Could you check a few things on this model? Use its own coordinates, in mm. A direction names the side the tool comes from. Round coordinates to 2 decimals unless told otherwise and drop trailing zeros. Loops run counter-clockwise (first coordinate to the right, second up) from the corner with the lowest first, then second, coordinate; pieces in that order, holes last. Notation, with made-up numbers: M 31.25,-29.75 L 87.25,-29.75 A25 ccw 87.25,-9.75 Z; hole C 87.5,81.25 d10. An arc over 180 degrees is marked long. Answer in a Markdown table with one row per item.
```python
from build123d import *

# Parameters (mm, degrees)
SKETCH_1_R      = 1.525
SKETCH_1_R_2    = 2.5
SKETCH_1_R_3    = 1.625
SKETCH_1_W      = 12.5
SKETCH_1_H      = 5
SKETCH_1_W_2    = 40
SKETCH_1_H_2    = 20
EXTRUDE_1_DEPTH = 5
FILLET_1_R      = 5


with BuildPart() as part:
    # 草图1 → 凸台-拉伸1 (new body)
    with BuildSketch(Plane(origin=(0, 0, 0), x_dir=(1, 0, 0), z_dir=(0, 1, 0))):
        with BuildLine():
            Line((41.868178549, 31.675), (158.5, 31.675))
            Line((158.5, 31.675), (158.5, -31.675))
            Line((158.5, -31.675), (41.868178549, -31.675))
            ThreePointArc((41.868178549, -31.675), (-52.5, 0), (41.868178549, 31.675))
        make_face()
        with Locations(Location((-33.55358156, 33.720895004, 0), (0, 0, 270))):
            Circle(SKETCH_1_R, mode=Mode.SUBTRACT)
        with Locations(Location((0, 0, 0), (0, 0, 270))):
            Circle(SKETCH_1_R_2, mode=Mode.SUBTRACT)
        with Locations(Location((82.254, 18.675, 0), (0, 0, 270))):
            Circle(SKETCH_1_R_3, mode=Mode.SUBTRACT)
        with Locations(Location((82.254, -8.825, 0), (0, 0, 270))):
            Circle(SKETCH_1_R_3, mode=Mode.SUBTRACT)
        with Locations(Location((135, 24.425, 0), (0, 0, 270))):
            Circle(SKETCH_1_R_3, mode=Mode.SUBTRACT)
        with Locations(Location((135, -24.425, 0), (0, 0, 90))):
            Circle(SKETCH_1_R_3, mode=Mode.SUBTRACT)
        with Locations(Location((33.720895004, 33.55358156, 0), (0, 0, 270))):
            Circle(SKETCH_1_R, mode=Mode.SUBTRACT)
        with Locations(Location((33.55358156, -33.720895004, 0), (0, 0, 270))):
            Circle(SKETCH_1_R, mode=Mode.SUBTRACT)
        with Locations(Location((-33.720895004, -33.55358156, 0), (0, 0, 270))):
            Circle(SKETCH_1_R, mode=Mode.SUBTRACT)
        with Locations((23.75, -20)):
            Rectangle(SKETCH_1_W, SKETCH_1_H, mode=Mode.SUBTRACT)
        with Locations((-23.75, 20)):
            Rectangle(SKETCH_1_W, SKETCH_1_H, mode=Mode.SUBTRACT)
        with Locations((0, 20)):
            Rectangle(SKETCH_1_W, SKETCH_1_H, mode=Mode.SUBTRACT)
        with Locations((23.75, 20)):
            Rectangle(SKETCH_1_W, SKETCH_1_H, mode=Mode.SUBTRACT)
        with Locations((0, -20)):
            Rectangle(SKETCH_1_W, SKETCH_1_H, mode=Mode.SUBTRACT)
        with Locations((-23.75, -20)):
            Rectangle(SKETCH_1_W, SKETCH_1_H, mode=Mode.SUBTRACT)
        with BuildLine():
            Line((-10, -30.25), (10, -30.25))
            ThreePointArc((10, -30.25), (15, -35.25), (10, -40.25))
            Line((10, -40.25), (-10, -40.25))
            ThreePointArc((-10, -40.25), (-15, -35.25), (-10, -30.25))
        make_face(mode=Mode.SUBTRACT)
        with BuildLine():
            Line((-10, 40.25), (10, 40.25))
            ThreePointArc((10, 40.25), (15, 35.25), (10, 30.25))
            Line((10, 30.25), (-10, 30.25))
            ThreePointArc((-10, 30.25), (-15, 35.25), (-10, 40.25))
        make_face(mode=Mode.SUBTRACT)
        with BuildLine():
            Line((48.183761531, 20.125053296), (48.183761531, -20.125053296))
            ThreePointArc((48.183761531, -20.125053296), (50, -21.941291765), (51.816238469, -20.125053296))
            Line((51.816238469, -20.125053296), (51.816238469, 20.125053296))
            ThreePointArc((51.816238469, 20.125053296), (50, 21.941291765), (48.183761531, 20.125053296))
        make_face(mode=Mode.SUBTRACT)
        with BuildLine():
            Line((68.183761531, 20.125053296), (68.183761531, -20.125053296))
            ThreePointArc((68.183761531, -20.125053296), (70, -21.941291765), (71.816238469, -20.125053296))
            Line((71.816238469, -20.125053296), (71.816238469, 20.125053296))
            ThreePointArc((71.816238469, 20.125053296), (70, 21.941291765), (68.183761531, 20.125053296))
        make_face(mode=Mode.SUBTRACT)
        with Locations((114.25, 0)):
            Rectangle(SKETCH_1_W_2, SKETCH_1_H_2, mode=Mode.SUBTRACT)
    extrude(amount=EXTRUDE_1_DEPTH)

    # 圆角1
    fillet_1_edges = [part.edges().sort_by_distance(p)[0] for p in [
        (94.25, 2.5, -10),
        (94.25, 2.5, 10),
        (134.25, 2.5, 10),
        (134.25, 2.5, -10),
        (41.868178549, 2.5, -31.675),
        (158.5, 2.5, -31.675),
        (158.5, 2.5, 31.675),
        (41.868178549, 2.5, 31.675),
    ]]
    fillet(fillet_1_edges, radius=FILLET_1_R)


solid = part.part
```
1) I want a section at A-A, the plane x = 104. Please give me the cut outline in (y, z) (3 decimals), plus the area to 3 significant figures.
Computed:
| item | result |
|---|---|
| outline | M 0,-31.675 L 5,-31.675 L 5,-10 L 0,-10 Z; M 0,10 L 5,10 L 5,31.675 L 0,31.675 Z |
| area | 217 mm² |
2) If we mould it in two halves opening along X, with no side actions, what happens to faces 4 (the face through (-52.47, 2.46, 1.8)), 5 (the face through (15, 2.46, -35.36)), 6 (the face through (100, 2, 31.675)), 7 (the face through (156.996, 2.535, -30.249))? For each: released by +X, released by -X, zero draft, split by the parting line, or undercut.
Computed:
| item | result |
|---|---|
| face 4 | split by the parting line |
| face 5 | undercut |
| face 6 | zero draft |
| face 7 | released by +X |
3) I want a section at D-D, the plane y = 3.65. State how many separate pieces and enclosed holes the cut face has, plus the area to 3 significant figures.
Computed:
| item | result |
|---|---|
| separate pieces | 1 |
| enclosed holes | 20 |
| area | 13,500 mm² |
4) Which directions (+Z, -Z, +X, -X, +Y, -Y) give clear straight access to the entire face, cutting with the end or side of a thin tool? Please do faces 1 (the face through (98, 2, -31.675)), 2 (the face through (-6.25, 2, 20)), 3 (the face through (42.13, 2.535, 32.163)).
Computed:
| item | result |
|---|---|
| face 1 | -Z, +X, +Y, -Y |
| face 2 | +Y, -Y |
| face 3 | +Z, +X, +Y, -Y |
5) Will these pins go through, and if not, where does the flat tip stop? P1, Ø2.5, axis at y = 3.5, z = -20, coming from the -X side; P2, Ø2.5, axis at x = 23.5, y = 3.5, coming from the +Z side; P3, Ø1, axis at x = -27.5, y = 3, coming from the +Z side (3 decimals); P4, Ø1.5, axis at x = 46.5, z = 20.5, coming from the -Y side.
Computed:
| item | result |
|---|---|
| P1 | stops at x = -49.04 |
| P2 | stops at z = 47.55 |
| P3 | stops at z = 45.025 |
| P4 | stops at y = 0 |
6) I want a section at C-C, the plane x = 0. Please give me the cut outline in (y, z).
Computed:
| item | result |
|---|---|
| outline | M 0,-52.5 L 5,-52.5 L 5,-40.25 L 0,-40.25 Z; M 0,-30.25 L 5,-30.25 L 5,-22.5 L 0,-22.5 Z; M 0,-17.5 L 5,-17.5 L 5,-2.5 L 0,-2.5 Z; M 0,2.5 L 5,2.5 L 5,17.5 L 0,17.5 Z; M 0,22.5 L 5,22.5 L 5,30.25 L 0,30.25 Z; M 0,40.25 L 5,40.25 L 5,52.5 L 0,52.5 Z |
7) I want a section at B-B, the plane z = 0. Please give me the cut outline in (x, y), plus the area to 3 significant figures.
Computed:
| item | result |
|---|---|
| outline | M -52.5,0 L -2.5,0 L -2.5,5 L -52.5,5 Z; M 2.5,0 L 48.18,0 L 48.18,5 L 2.5,5 Z; M 51.82,0 L 68.18,0 L 68.18,5 L 51.82,5 Z; M 71.82,0 L 94.25,0 L 94.25,5 L 71.82,5 Z; M 134.25,0 L 158.5,0 L 158.5,5 L 134.25,5 Z |
| area | 794 mm² |
8) I need wall thicknesses on line 1 (X direction, y = 1.7, z = -34.5); line 2 (Z direction, x = 9, y = 3.5); line 3 (X direction, y = 0.75, z = -15). Which ranges of each line are inside material? Lowest first, please.
Computed:
| item | result |
|---|---|
| line 1 | x = -39.57 to -34.86, -32.24 to -14.94, 14.94 to 32.53, 34.92 to 39.57 |
| line 2 | z = -51.72 to -40.25, -30.25 to 30.25, 40.25 to 51.72 |
| line 3 | x = -50.31 to 48.18, 51.82 to 68.18, 71.82 to 158.5 |
